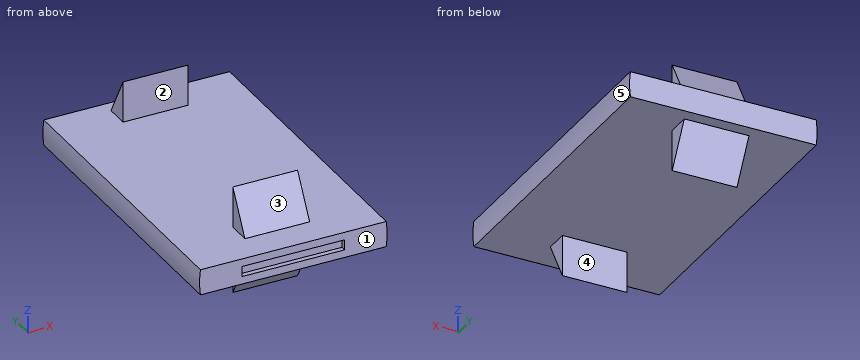
```python
from build123d import *

# Parameters (mm, degrees)
SKETCH1_W           = 99.06
SKETCH1_H           = 360.68
BOSS_EXTRUDE1_DEPTH = 12.7
SKETCH3_W           = 32.004
SKETCH3_H           = 11.43
BOSS_EXTRUDE3_DEPTH = 20.32
SKETCH2_W           = 55.88
SKETCH2_H           = 12.7
BOSS_EXTRUDE4_DEPTH = 7.62
CUT_EXTRUDE2_DEPTH  = 38.1
SKETCH6_W           = 50.8
SKETCH6_H           = 5.08
CUT_EXTRUDE3_DEPTH  = 2.54
SKETCH7_R           = 50.8
SKETCH7_R_2         = 46.355
CUT_EXTRUDE4_DEPTH  = 366.559302576
SKETCH9_W           = 155.282238602
SKETCH9_H           = 226.847096393
CUT_EXTRUDE9_DEPTH  = 25.4


with BuildPart() as part:
    # Sketch1 → Boss-Extrude1 (new body)
    with BuildSketch(Plane.XY):
        Rectangle(SKETCH1_W, SKETCH1_H)
    extrude(amount=BOSS_EXTRUDE1_DEPTH)

    # Sketch3 → Boss-Extrude3 (add)
    with BuildSketch(Plane(origin=(0, 0, 0), x_dir=(-1, 0, 0), z_dir=(0, 0, -1))):
        with Locations((0, -43.815)):
            Rectangle(SKETCH3_W, SKETCH3_H)
        with Locations((0, -159.385)):
            Rectangle(SKETCH3_W, SKETCH3_H)
    boss_extrude3 = extrude(amount=BOSS_EXTRUDE3_DEPTH)

    # Sketch2 → Boss-Extrude4 (add, symmetric)
    with BuildSketch(Plane.XY.offset(12.7)):
        with Locations((0, 171.45)):
            Rectangle(SKETCH2_W, SKETCH2_H)
        with Locations((0, -19.05)):
            Rectangle(SKETCH2_W, SKETCH2_H)
    extrude(amount=BOSS_EXTRUDE4_DEPTH, both=True)

    # Mirror1: Boss-Extrude3 across plane
    add(boss_extrude3.mirror(Plane.XY.offset(6.35)))

    # Sketch5 → Cut-Extrude2 (cut, symmetric)
    with BuildSketch(Plane(origin=(0, 0, 0), x_dir=(0, 0, -1), z_dir=(1, 0, 0))):
        Polygon((20.32, -153.67), (0, -165.1), (20.32, -165.1), align=None)
        Polygon((-33.02, -153.67), (-12.7, -165.1), (-33.02, -165.1), align=None)
        Polygon((-33.02, -49.53), (-33.02, -38.1), (-12.7, -38.1), align=None)
        Polygon((20.32, -49.53), (0, -38.1), (20.32, -38.1), align=None)
        Polygon((-12.7, 177.8), (-20.32, 165.1), (-20.32, 177.8), align=None)
        Polygon((-20.32, -12.7), (-12.7, -25.4), (-20.32, -25.4), align=None)
    extrude(amount=CUT_EXTRUDE2_DEPTH, both=True, mode=Mode.SUBTRACT)

    # Sketch6 → Cut-Extrude3 (cut)
    with BuildSketch(Plane(origin=(0, 180.34, 0), x_dir=(1, 0, 0), z_dir=(0, 1, 0))):
        with Locations((0, -6.35)):
            Rectangle(SKETCH6_W, SKETCH6_H)
    cut_extrude3 = extrude(amount=-CUT_EXTRUDE3_DEPTH, mode=Mode.SUBTRACT)

    # Mirror2: Cut-Extrude3 across plane
    add(cut_extrude3.mirror(Plane.ZX), mode=Mode.SUBTRACT)

    # Sketch7 → Cut-Extrude4 (cut, through all)
    with BuildSketch(Plane(origin=(0, 180.34, 0), x_dir=(1, 0, 0), z_dir=(0, 1, 0))):
        with Locations((0, -6.35)):
            Circle(SKETCH7_R)
        with Locations((0, -6.35)):
            Circle(SKETCH7_R_2, mode=Mode.SUBTRACT)
    extrude(amount=-CUT_EXTRUDE4_DEPTH, mode=Mode.SUBTRACT)

    # Sketch9 → Cut-Extrude9 (cut, symmetric)
    with BuildSketch(Plane.XY):
        with Locations((0, 81.673548197)):
            Rectangle(SKETCH9_W, SKETCH9_H)
    extrude(amount=CUT_EXTRUDE9_DEPTH, both=True, mode=Mode.SUBTRACT)


solid = part.part
```
Here's how the part is built. I have some questions about the finished solid (model axes, mm). Face numbers are marked on the shaded views. A direction names the side the tool comes from. Round coordinates to 2 decimals unless told otherwise and drop trailing zeros. Order: outer loops, then holes, each group sorted by start corner. A loop starts at its lowest first (then second) coordinate and runs counter-clockwise, first axis right, second up. Notation, with made-up numbers: M 10.25,-29.5 L 27.25,-29.5 A18 ccw 27.25,-23.5 Z; hole C 45.5,23.25 d3. An arc over 180 degrees is marked long. Answer as CSV lines item,"result".
Item 1: Which directions (+Z, -Z, +X, -X, +Y, -Y) give clear straight access to the entire face, cutting with the end or side of a thin tool? Please do the marked faces 1 and 2.
From the geometry:
face 1,"+Z, -Z, +X, -X, -Y"
face 2,"+Z, +X, -X"
Item 2: Imagine slicing it at B-B on x = -18. List the corners of the cut face in (y, z) for me, and give its area (3 significant figures).
From the geometry:
outline,"M -180.34,0 L -31.75,0 L -31.75,12.7 L -180.34,12.7 L -180.34,8.89 L -177.8,8.89 L -177.8,3.81 L -180.34,3.81 Z"
area,"1,870 mm2"
Item 3: Imagine slicing it at A-A on z = 23.5. List the corners of the cut face in (x, y) for me (3 decimals).
From the geometry:
outline,"M -16.002,-159.025 L 16.002,-159.025 L 16.002,-153.67 L -16.002,-153.67 Z; M -16.002,-49.53 L 16.002,-49.53 L 16.002,-44.175 L -16.002,-44.175 Z"
Item 4: Imagine slicing it at D-D on z = 30. List the corners of the cut face in (x, y) for me, and give its area (3 significant figures).
From the geometry:
outline,"M -16,-155.37 L 16,-155.37 L 16,-153.67 L -16,-153.67 Z; M -16,-49.53 L 16,-49.53 L 16,-47.83 L -16,-47.83 Z"
area,"109 mm2"
Item 5: Imagine slicing it at C-C on y = -47. List the corners of the cut face in (x, z) for me (3 decimals), and give its area (3 significant figures).
From the geometry:
outline,"M -45.918,0 L -16.002,0 L -16.002,-15.822 L 16.002,-15.822 L 16.002,0 L 45.918,0 A46.355 ccw 45.918,12.7 L 16.002,12.7 L 16.002,28.522 L -16.002,28.522 L -16.002,12.7 L -45.918,12.7 A46.355 ccw Z"
area,"2,190 mm2"
Item 6: We'd pull the mould along Y, two halves only. Please class the marked faces 3, 4 and 5: +Y half, -Y half, draft (parallel to the pull), parting line (faces both ways), or undercut.
From the geometry:
face 3,"-Y half"
face 4,"undercut"
face 5,"draft"
Item 7: Please list where these lines run through material, in increasing order: L1, parallel to Z at x = -1, y = -89; L2, parallel to X at y = -56.5, z = 6; L3, parallel to Y at x = -4, z = 30. Write a range as [from, to].
From the geometry:
L1,"[0, 12.7]"
L2,"[-46.35, 46.35]"
L3,"[-155.37, -153.67], [-49.53, -47.83]"
Item 8: For pin 1 (5 mm diameter, centred on y = -134.5, z = 12.5, fed in from +X); pin 2 (0.8 mm diameter, centred on y = -179, z = 7, fed in from +X); pin 3 (2 mm diameter, centred on x = 10.5, z = -13, fed in from +Y); pin 4 (10 mm diameter, centred on y = -113.5, z = -6, fed in from +X), each with a flat end and sliding along its axis, tell me the tip position at first contact or that it passes through.
From the geometry:
pin 1,"x = 46.21"
pin 2,"x = 46.35"
pin 3,"y = -44.85"
pin 4,"through"
